```python
from build123d import *

# Parameters (mm, degrees)
BOSS_EXTRUDE1_DEPTH                                 = 2.54
SKETCH2_R                                           = 3.175
BOSS_EXTRUDE2_DEPTH                                 = 15
CBORE_FOR_00_BINDING_HEAD_MACHINE_SCREW_D           = 3.048
CBORE_FOR_00_BINDING_HEAD_MACHINE_SCREW_CBORE_D     = 5.715
CBORE_FOR_00_BINDING_HEAD_MACHINE_SCREW_CBORE_DEPTH = 5.08
CBORE_FOR_00_BINDING_HEAD_MACHINE_S_2_D             = 3.048
CBORE_FOR_00_BINDING_HEAD_MACHINE_S_2_CBORE_D       = 5.715
CBORE_FOR_00_BINDING_HEAD_MACHINE_S_2_CBORE_DEPTH   = 5.08


with BuildPart() as part:
    # Sketch1 → Boss-Extrude1 (new body)
    with BuildSketch(Plane.XZ.offset(14.999999665)):
        with BuildLine():
            ThreePointArc((-118.732237126, 41.291635073), (-119.799942246, 44.449254661), (-118.68060362, 47.588942022))
            Line((-118.68060362, 47.588942022), (-98.069142774, 73.248424617))
            ThreePointArc((-98.069142774, 73.248424617), (-95.812668617, 80.026590118), (-101.944824249, 76.361638481))
            Line((-101.944824249, 76.361638481), (-120.087244283, 52.215986296))
            ThreePointArc((-120.087244283, 52.215986296), (-124.066396106, 50.188221558), (-128.109054429, 52.086218591))
            Line((-128.109054429, 52.086218591), (-147.547470085, 76.285361579))
            ThreePointArc((-147.547470085, 76.285361579), (-153.664676639, 80.026590118), (-151.33049651, 73.246574622))
            Line((-151.33049651, 73.246574622), (-130.017313744, 47.964682708))
            ThreePointArc((-130.017313744, 47.964682708), (-128.821664975, 44.750582309), (-129.940817748, 41.509052665))
            Line((-129.940817748, 41.509052665), (-151.408202483, 14.784019002))
            ThreePointArc((-151.408202483, 14.784019002), (-153.664676639, 8.0058535), (-147.532521008, 11.670805138))
            Line((-147.532521008, 11.670805138), (-128.34443149, 35.558313777))
            ThreePointArc((-128.34443149, 35.558313777), (-124.342289826, 37.456804622), (-120.37181674, 35.49294392))
            Line((-120.37181674, 35.49294392), (-101.929875172, 11.74708204))
            ThreePointArc((-101.929875172, 11.74708204), (-95.812668617, 8.0058535), (-98.146848747, 14.785868997))
            Line((-98.146848747, 14.785868997), (-118.732237126, 41.291635073))
        make_face()
    extrude(amount=BOSS_EXTRUDE1_DEPTH)

    # Sketch2 → Boss-Extrude2 (add)
    with BuildSketch(Plane(origin=(0, -14.999999665, 0), x_dir=(1, 0, 0), z_dir=(0, 1, 0))):
        with Locations((-98.19867242, -10.976221467)):
            Circle(SKETCH2_R)
        with Locations((-151.278672837, -10.976221467)):
            Circle(SKETCH2_R)
        with Locations((-151.278672837, -77.056222152)):
            Circle(SKETCH2_R)
        with Locations((-98.19867242, -77.056222152)):
            Circle(SKETCH2_R)
    extrude(amount=BOSS_EXTRUDE2_DEPTH)

    # CBORE for _00 Binding Head Machine Screw (through all)
    with Locations(Plane(origin=(0, -17.539999665, 0), x_dir=(-1, 0, 0), z_dir=(0, -1, 0))):
        with Locations((151.278672837, -10.976221467)):
            CounterBoreHole(CBORE_FOR_00_BINDING_HEAD_MACHINE_SCREW_D / 2, CBORE_FOR_00_BINDING_HEAD_MACHINE_SCREW_CBORE_D / 2, CBORE_FOR_00_BINDING_HEAD_MACHINE_SCREW_CBORE_DEPTH)

    # CBORE for _00 Binding Head Machine S 2 (through all)
    with Locations(Plane(origin=(0, -17.539999665, 0), x_dir=(-1, 0, 0), z_dir=(0, -1, 0))):
        with Locations((98.19867242, -10.976221467), (98.19867242, -77.056222152), (151.278672837, -77.056222152)):
            CounterBoreHole(CBORE_FOR_00_BINDING_HEAD_MACHINE_S_2_D / 2, CBORE_FOR_00_BINDING_HEAD_MACHINE_S_2_CBORE_D / 2, CBORE_FOR_00_BINDING_HEAD_MACHINE_S_2_CBORE_DEPTH)


solid = part.part
```
Part model, mm, in its own coordinate system. A direction names the side the tool comes from. Give positions to 0.01 mm unless a question says otherwise; leave off trailing zeros. Order: outer loops, then holes, each group sorted by start corner. A loop starts at its lowest first (then second) coordinate and runs counter-clockwise, first axis right, second up. Notation, with made-up numbers: M 23,24 L 61,24 A25 ccw 61,60 Z; hole C 80,83.5 d6. An arc over 180 degrees is marked long. Use a Markdown table: item, result. Add a question column.
(1) Drop flat-ended pins along their axis: P1, Ø1.5, axis at x = -136.5, z = 52.5, coming from the -Y side; P2, Ø3, axis at x = -149, y = -11, coming from the +Z side; P3, Ø1.7, axis at x = -152.5, z = 10, coming from the -Y side; P4, Ø4, axis at x = -142.5, y = -13.5, coming from the -Z side. Give the stop position or say it passes through.
(2) Saw through at A-A, the plane x = -135. Give the cut face in (y, z).
(3) Mould opens along X. For faces 1 (the face through (-100.924, -15.036, 10.118)), 2 (the face through (-108.295, -16.252, 27.853)), 3 (the face through (-140.82, -16.25, 60.78)) say: +X half, -X half, draft (parallel to the pull), parting line (faces both ways), or undercut.
(4) Saw through at D-D, the plane y = -5.25. Give the cut face in (x, z) (3 decimals), and give its area (3 significant figures).
(5) Saw through at C-C, the plane z = 55. Give the cut face in (x, y), and give its area (3 significant figures).
(6) Probe line 1 along X through (y, z) = (-15.25, 74.5); line 2 along Z through (x, y) = (-151, -10.5); line 3 along Z through (x, y) = (-97, -10.5). List the from-to ranges inside material, lowest first. Write a range as [from, to].
(7) 3-axis set-ups, long thin cutter, end or side, ignore diameter. For faces 4 (the face through (-108.52, -16.25, 60.24)), 5 (the face through (-153, 0, 12)), 6 (the face through (-153.92, -15.04, 78.15)), 7 (the face through (-151.967, -7.605, 80.156)): which of +Z, -Z, +X, -X, +Y, -Y reach the whole face in a straight line?
(8) Saw through at B-B, the plane y = -14. Give the number of separate pieces and of enclosed holes in the cut face, and give its area (3 significant figures).
Answer key:
| question | item | result |
|---|---|---|
| 1 | P1 | through |
| 1 | P2 | z = 80.13 |
| 1 | P3 | y = -12.46 |
| 1 | P4 | z = 16.29 |
| 2 | outline | M -17.54,27.27 L -15,27.27 L -15,35.21 L -17.54,35.21 Z; M -17.54,53.88 L -15,53.88 L -15,60.66 L -17.54,60.66 Z |
| 3 | face 1 | undercut |
| 3 | face 2 | +X half |
| 3 | face 3 | -X half |
| 4 | outline | C -151.279,10.976 d6.35; C -151.279,77.056 d6.35; C -98.199,10.976 d6.35; C -98.199,77.056 d6.35; hole C -151.279,10.976 d3.048; hole C -151.279,77.056 d3.048; hole C -98.199,10.976 d3.048; hole C -98.199,77.056 d3.048 |
| 4 | area | 97.5 mm^2 |
| 5 | outline | M -135.95,-17.54 L -130.45,-17.54 L -130.45,-15 L -135.95,-15 Z; M -118,-17.54 L -112.73,-17.54 L -112.73,-15 L -118,-15 Z |
| 5 | area | 27.3 mm^2 |
| 6 | line 1 | [-154.1, -152.56], [-150, -146.11], [-103.34, -99.48], [-96.92, -95.37] |
| 6 | line 2 | [7.81, 9.48], [12.47, 14.14], [73.89, 75.56], [78.55, 80.22] |
| 6 | line 3 | [8.04, 10.04], [11.92, 13.92], [74.12, 76.12], [78, 80] |
| 7 | face 4 | +X, +Y, -Y |
| 7 | face 5 | +Z, -Z, +X, -X, +Y |
| 7 | face 6 | -Y |
| 7 | face 7 | +Y |
| 8 | separate pieces | 4 |
| 8 | enclosed holes | 4 |
| 8 | area | 24.1 mm^2 |
